For this review, take the finished solid that the model builds, in its own axes (mm). A direction names the side the tool comes from. Give positions to 0.01 mm unless a question says otherwise; leave off trailing zeros. Order: outer loops, then holes, each group sorted by start corner. A loop starts at its lowest first (then second) coordinate and runs counter-clockwise, first axis right, second up.
from build123d import *

# Parameters (mm, degrees)
BOSS_EXTRUDE4_DEPTH      = 2.4
BOSS_EXTRUDE4_2_DEPTH    = 2.4
BOSS_EXTRUDE4_3_DEPTH    = 2.4
BOSS_EXTRUDE4_4_DEPTH    = 2.4
BOSS_EXTRUDE5_DEPTH      = 7
SKETCH2_R                = 1.499999999999997
BOSS_EXTRUDE8_DEPTH      = 0.8
SKETCH3_R                = 1.5000000000000007
BOSS_EXTRUDE9_DEPTH      = 0.8
SKETCH4_R                = 1.6999999999999995
CUT_EXTRUDE3_DEPTH       = 1.2
SKETCH5_R                = 1.6999999999999995
CUT_EXTRUDE4_DEPTH       = 1.2
CHAMFER4_SIZE            = 2
CUT_EXTRUDE7_REACH       = 33.329
SKETCH8_R                = 0.3999999999999905
SKETCH8_R_2              = 0.4000000000000032
CUT_EXTRUDE10_DEPTH      = 2
CHAMFER6_SIZE            = 0.8
CUT_EXTRUDE11_DEPTH      = 10
CUT_EXTRUDE11_DEPTH_BACK = 1.4
BOSS_EXTRUDE10_DEPTH     = 3.6
CHAMFER8_SIZE            = 2.6


with BuildPart() as part:
    # Sketch1 → Boss-Extrude4 (new body)
    with BuildSketch(Plane(origin=(0, 0, 0), x_dir=(1, 0, 0), z_dir=(0, 1, 0))):
        Polygon((-6.430686748297487, -2.000308799271804), (-6.118186748297487, -4.480700653394857), (-2.1999999999999993, -3.9870555235708633), (-2.1999999999999997, -1.4672923701760037), align=None)
    extrude(amount=BOSS_EXTRUDE4_DEPTH)



with BuildPart() as body_2:
    # Sketch1 → Boss-Extrude4 2 (new body)
    with BuildSketch(Plane(origin=(0, 0, 0), x_dir=(1, 0, 0), z_dir=(0, 1, 0))):
        Polygon((-10.000000000000064, 2.4499999999999993), (-9.689951018234682, -0.01093750000000027), (-6.316618096627332, 0.41406249999999967), (-6.626667078392713, 2.8750000000000004), align=None)
    extrude(amount=BOSS_EXTRUDE4_2_DEPTH)


with BuildPart() as body_3:
    # Sketch1 → Boss-Extrude4 3 (new body)
    with BuildSketch(Plane(origin=(0, 0, 0), x_dir=(1, 0, 0), z_dir=(0, 1, 0))):
        Polygon((5.961321581281771, -0.4390625000000079), (2.200000000000001, -0.9129444764291388), (2.200000000000001, -3.432707629823996), (6.273821581281774, -2.919454354123064), align=None)
    extrude(amount=BOSS_EXTRUDE4_3_DEPTH)


with BuildPart() as body_4:
    # Sketch1 → Boss-Extrude4 4 (new body)
    with BuildSketch(Plane(origin=(0, 0, 0), x_dir=(1, 0, 0), z_dir=(0, 1, 0))):
        Polygon((6.159752929611616, 4.485937500000006), (6.469801911377001, 2.025000000000001), (9.843134832984354, 2.4499999999999993), (9.533085851218969, 4.910937500000012), align=None)
    extrude(amount=BOSS_EXTRUDE4_4_DEPTH)


with BuildPart() as part_1:
    add(part.part)

    add(body_2.part)  # Boss-Extrude5 merges body 2

    add(body_3.part)  # Boss-Extrude5 merges body 3

    add(body_4.part)  # Boss-Extrude5 merges body 4
    # Sketch1<8> → Boss-Extrude5 (add)
    with BuildSketch(Plane(origin=(0, 0, 0), x_dir=(1, 0, 0), z_dir=(0, 1, 0))):
        Polygon((-20, -0.05000000000000027), (-20, -2.45), (-12, -2.4499999999999997), (-10.000000000000064, -2.4499999999999997), (-6.430686748297488, -2.000308799271796), (-2.5125, -1.5066636694477982), (-2.1999999999999993, -1.467292370176004), (-2.1999999999999997, 0.9327076298239989), (-6.316618096627332, 0.41406249999999967), (-9.689951018234682, -0.01093750000000025), (-10.000000000000064, -0.05000000000000029), (-12, -0.05000000000000027), align=None)
        Polygon((2.2000000000000006, 1.487055523570866), (2.2000000000000006, -0.9129444764291423), (5.961321581281771, -0.4390625000000079), (9.687500000000064, 0.03039185412306233), (9.843134832984425, 0.05000000000000027), (12, 0.05000000000000013), (20, 0.05000000000000013), (20, 2.4499999999999997), (12, 2.4499999999999993), (9.843134832984353, 2.4499999999999993), (6.469801911376997, 2.024999999999999), (2.510048981765383, 1.526118023570866), align=None)
        Polygon((-2.1999999999999997, 0.9327076298239989), (-2.1999999999999997, -1.4672923701760037), (2.200000000000001, -0.9129444764291388), (2.2000000000000006, 1.487055523570866), align=None)
    extrude(amount=BOSS_EXTRUDE5_DEPTH)

    # Sketch2 → Boss-Extrude8 (add)
    with BuildSketch(Plane.XY.offset(2.4499999999999993)):
        with Locations(Location((-16.5, 3.4999999999999996, 0), (0, 0, 180))):
            Circle(SKETCH2_R)
    extrude(amount=BOSS_EXTRUDE8_DEPTH)

    # Sketch3 → Boss-Extrude9 (add)
    with BuildSketch(Plane.XY.offset(-0.05000000000000013)):
        with Locations(Location((16.5, 3.4999999999999996, 0), (0, 0, 180))):
            Circle(SKETCH3_R)
    extrude(amount=BOSS_EXTRUDE9_DEPTH)

    # Sketch4 → Cut-Extrude3 (cut)
    with BuildSketch(Plane(origin=(0, 0, 0.05000000000000041), x_dir=(-1, 0, -5e-17), z_dir=(5e-17, 0, -1))):
        with Locations((16.5, 3.4999999999999996)):
            Circle(SKETCH4_R)
    extrude(amount=-CUT_EXTRUDE3_DEPTH, mode=Mode.SUBTRACT)

    # Sketch5 → Cut-Extrude4 (cut)
    with BuildSketch(Plane(origin=(-1e-16, 0, -2.449999999999999), x_dir=(-1, 0, 5e-17), z_dir=(-5e-17, 0, -1))):
        with Locations((-16.5, 3.4999999999999996)):
            Circle(SKETCH5_R)
    extrude(amount=-CUT_EXTRUDE4_DEPTH, mode=Mode.SUBTRACT)

    # Chamfer4
    chamfer4_edges = [part_1.edges().sort_by_distance(p)[0] for p in [
        (20, 7, -1.25),
        (-20, 7, 1.2500000000000002),
        (-20, 0, 1.2500000000000002),
        (20, 0, -1.25),
    ]]
    chamfer(chamfer4_edges, length=CHAMFER4_SIZE)

    # Cut-Extrude7: up to this face of the body (flat: up to its plane)
    cut_extrude7_end = Plane(part_1.part.faces().sort_by_distance((-9.844975509, 1.2, -1.21953125))[0])
    # Sketch8 → Cut-Extrude7 (cut, up to the picked face)
    with BuildSketch(Plane(origin=(9.99318385334905, 0, -1.2590228229384695), x_dir=(-0.12500000000000053, 0, -0.9921567416492215), z_dir=(0.9921567416492215, 0, -0.12500000000000053)), mode=Mode.PRIVATE) as cut_extrude7_sk1:
        with Locations((2.4807840170405906, 1.2000000000000017)):
            Circle(SKETCH8_R)
    cut_extrude7_tool1 = split(extrude(cut_extrude7_sk1.sketch, amount=-CUT_EXTRUDE7_REACH, mode=Mode.PRIVATE), bisect_by=cut_extrude7_end, keep=Keep.BOTH, mode=Mode.PRIVATE)
    # Sketch8 → Cut-Extrude7 (cut, up to the picked face)
    with BuildSketch(Plane(origin=(9.99318385334905, 0, -1.2590228229384695), x_dir=(-0.12500000000000053, 0, -0.9921567416492215), z_dir=(0.9921567416492215, 0, -0.12500000000000053)), mode=Mode.PRIVATE) as cut_extrude7_sk2:
        with Locations((-2.4807840170405973, 1.200000000000001)):
            Circle(SKETCH8_R_2)
    cut_extrude7_tool2 = split(extrude(cut_extrude7_sk2.sketch, amount=-CUT_EXTRUDE7_REACH, mode=Mode.PRIVATE), bisect_by=cut_extrude7_end, keep=Keep.BOTH, mode=Mode.PRIVATE)
    add(cut_extrude7_tool1.solids().sort_by(Axis((9.683086, 1.2, -3.720349), (-0.9921567416492215, 0, 0.12500000000000053)))[0], mode=Mode.SUBTRACT)
    add(cut_extrude7_tool2.solids().sort_by(Axis((10.303282, 1.2, 1.202304), (-0.9921567416492215, 0, 0.12500000000000053)))[0], mode=Mode.SUBTRACT)

    # Sketch1<10> → Cut-Extrude10 (cut)
    with BuildSketch(Plane(origin=(0, 0, 0), x_dir=(1, 0, 0), z_dir=(0, 1, 0))):
        Polygon((-2.1999999999999997, 0.9327076298239989), (-2.1999999999999997, -1.4672923701760037), (2.200000000000001, -0.9129444764291388), (2.2000000000000006, 1.487055523570866), align=None)
        Polygon((-2.2, 3.432707629823986), (-2.1999999999999997, 0.9327076298239989), (2.200000000000001, 1.487055523570866), (2.2, 3.987055523570867), align=None)
        Polygon((2.200000000000001, -0.9129444764291388), (-2.1999999999999993, -1.467292370176004), (-2.1999999999999993, -3.9870555235708607), (2.200000000000003, -3.432707629823997), align=None)
    extrude(amount=CUT_EXTRUDE10_DEPTH, mode=Mode.SUBTRACT)

    # Chamfer6
    chamfer6_edges = [part_1.edges().sort_by_distance(p)[0] for p in [
        (4.080660790640886, 2.4, 0.6760034882145733),
        (-4.315343374148743, 2.4, 1.7338005847239037),
        (-4.159093374148743, 0, 4.233878088482863),
        (-4.159093374148743, 2.4, 4.233878088482863),
        (7.846419390415299, 2.4, -4.698437499999993),
        (8.156468372180676, 2.4, -2.237499999999999),
        (7.846419390415299, 0, -4.698437499999993),
        (4.236910790640888, 2.4, 3.1760809919735298),
        (-8.313333539196389, 2.4, -2.6624999999999988),
        (-8.003284557431007, 2.4, -0.20156249999999976),
        (-8.313333539196389, 0, -2.6624999999999988),
        (4.236910790640888, 0, 3.1760809919735298),
    ]]
    chamfer(chamfer6_edges, length=CHAMFER6_SIZE)

    # Sketch9 → Cut-Extrude11 (cut, two sides: drawn at the far end of the back side and taken through both)
    with BuildSketch(Plane(origin=(0, 2.4, 0), x_dir=(1, 0, 0), z_dir=(0, 1, 0)).offset(-CUT_EXTRUDE11_DEPTH_BACK)):
        Polygon((-9.900000000000063, 1.6562746066806198), (-9.789951018234682, 0.7827878933193786), (-8.599362928255616, 0.9327878933193787), (-8.709411910020998, 1.8062746066806201), align=None)
        Polygon((-2.1999999999999993, -2.2736165792623466), (-3.390588089979065, -2.423616579262345), (-3.2780880899790614, -3.3165576467466713), (-2.087499999999996, -3.1665576467466714), align=None)
        Polygon((2.200000000000001, -2.626383420737649), (2.087499999999998, -1.733442353253328), (3.278088089979064, -1.5834423532533284), (3.3905880899790666, -2.47638342073765), align=None)
        Polygon((9.633085851218974, 4.117212106680604), (8.442497761239908, 3.967212106680604), (8.552546743005287, 3.0937253933193816), (9.743134832984353, 3.2437253933193815), align=None)
    extrude(amount=CUT_EXTRUDE11_DEPTH + CUT_EXTRUDE11_DEPTH_BACK, mode=Mode.SUBTRACT)

    # Sketch10 → Boss-Extrude10 (add)
    with BuildSketch(Plane(origin=(0, 6.999999999999999, 0), x_dir=(1, 0, 0), z_dir=(0, 1, 0))):
        Polygon((9.121272136324666, 4.979607528287985), (3.168331686429335, 4.22960752828798), (3.493331686429336, 1.6499999999999986), (9.446272136324666, 2.4000000000000035), align=None)
        Polygon((-9.618088321575, 2.6186700282879727), (-9.293088321574997, 0.03906249999999938), (-3.3401478716796675, 0.7890624999999998), (-3.665147871679668, 3.3686700282879767), align=None)
    extrude(amount=-BOSS_EXTRUDE10_DEPTH)

    # Chamfer8
    chamfer8_edges = [part_1.edges().sort_by_distance(p)[0] for p in [
        (-6.641618096627334, 3.399999999999999, -2.9936700282879745),
        (6.144801911377001, 3.399999999999999, -4.604607528287982),
    ]]
    chamfer(chamfer8_edges, length=CHAMFER8_SIZE - 0.0001)  # a hair under: the kernel refuses the full size


solid = part_1.part
1) We need section A-A on x = 16.5. Give the boundary of the cut face in (y, z), then the cut area to 3 significant figures.
Answer sheet:
outline: (0, -2.45) - (1.8, -2.45) - (1.8, -1.25) - (5.2, -1.25) - (5.2, -2.45) - (7, -2.45) - (7, -0.05) - (5, -0.05) - (5, 0.75) - (2, 0.75) - (2, -0.05) - (0, -0.05) - close
area: 15.1 mm2
2) Draft analysis for pull direction X (two halves, no side actions). For faces 1 (the face through (-0.217, 4.229, 1.217)), 2 (the face through (19, 1, -1)), 3 (the face through (-9.78, 0.87, -0.69)), state which applies: +X half, -X half, draft (parallel to the pull), parting line (faces both ways), or undercut.
Answer sheet:
face 1: undercut
face 2: +X half
face 3: -X half
3) Tool access review of faces 4 (the face through (-14, 3, 2.45)), 5 (the face through (-9.3, 1.69, -1.73)), 6 (the face through (4.108, 2.794, 1.081)): name each direction out of +Z, -Z, +X, -X, +Y, -Y from which nothing blocks a thin tool from reaching the whole face with its end or side.
Answer sheet:
face 4: +Z
face 5: none
face 6: +Z, +Y
4) Clearance check with flat-ended pins moving along their axes: pin 1 (3.5 mm diameter, centred on x = -17, y = 3, fed in from -Z); pin 2 (1 mm diameter, centred on x = 12, y = 2.5, fed in from +Z); pin 3 (2.5 mm diameter, centred on x = 17, y = 3.5, fed in from -Z). State where each tip first meets the part, or that it passes through.
Answer sheet:
pin 1: stops at z = 0.05
pin 2: stops at z = -0.05
pin 3: stops at z = -2.45
5) To check wall thickness, follow line 1 (Y direction, x = 16.5, z = -2.1); line 2 (Z direction, x = -17, y = 1); line 3 (X direction, y = 6.5, z = -2.25). State the ranges of each line that lie inside material, in increasing order.
Answer sheet:
line 1: y = 0 to 1.8, 5.2 to 7
line 2: z = 0.05 to 2.45
line 3: x = -9.57 to -3.52, 3.42 to 18.5
